Geometry check sheet. Reference: the model listing, model coordinates, mm. Face numbers are marked on the shaded views. A direction names the side the tool comes from. Round coordinates to 2 decimals unless told otherwise and drop trailing zeros. Loops run counter-clockwise (first coordinate to the right, second up) from the corner with the lowest first, then second, coordinate; pieces in that order, holes last.
```python
from build123d import *

# Parameters (mm, degrees)
SKETCH_1_R      = 118.75
EXTRUDE_1_DEPTH = 50
SKETCH_2_R      = 12.5
EXTRUDE_2_DEPTH = 10


with BuildPart() as part:
    # 草圖1 → 填料-伸長1 (new body)
    with BuildSketch(Plane(origin=(0, 0, 0), x_dir=(1, 0, 0), z_dir=(0, 1, 0))):
        Polygon((98.75, 128.75), (128.75, 98.75), (128.75, -98.75), (98.75, -128.75), (-98.75, -128.75), (-128.75, -98.75), (-128.75, 98.75), (-98.75, 128.75), align=None)
        with Locations(Location((0, 0, 0), (0, 0, 270))):
            Circle(SKETCH_1_R, mode=Mode.SUBTRACT)
    extrude(amount=EXTRUDE_1_DEPTH)

    # 草圖2 → 填料-伸長2 (add)
    with BuildSketch(Plane.XZ):
        Polygon((98.75, -128.75), (128.75, -98.75), (128.75, 98.75), (98.75, 128.75), (-98.75, 128.75), (-128.75, 98.75), (-128.75, -98.75), (-98.75, -128.75), align=None)
        with Locations(Location((0, 0, 0), (0, 0, 270))):
            Circle(SKETCH_2_R, mode=Mode.SUBTRACT)
    extrude(amount=-EXTRUDE_2_DEPTH)


solid = part.part
```
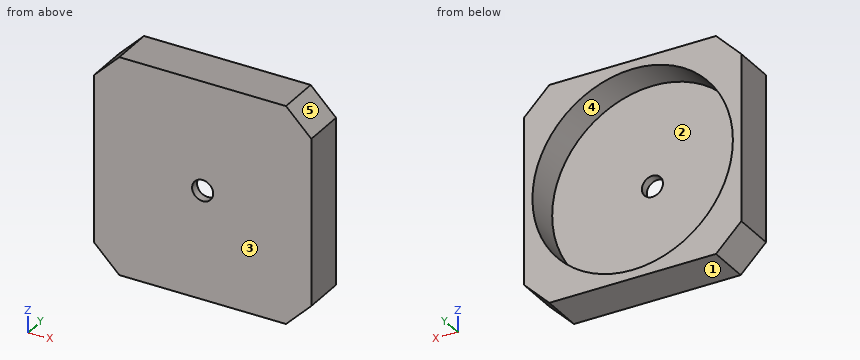
1) Sectioned sample at B-B, the plane z = 0. Record the cut outline in (x, y), then the cut area to 4 significant figures.
Report:
outline: (-128.75, 0) - (-12.5, 0) - (-12.5, 10) - (-118.75, 10) - (-118.75, 50) - (-128.75, 50) - close; (12.5, 0) - (128.75, 0) - (128.75, 50) - (118.75, 50) - (118.75, 10) - (12.5, 10) - close
area: 3,125 mm2
2) Mould release check, pull along Z, two halves, no side actions. Record for the marked faces 3, 4 and 5: +Z half, -Z half, draft (parallel to the pull), parting line (faces both ways), or undercut.
Report:
face 3: draft
face 4: undercut
face 5: +Z half
3) Sectioned sample at C-C, the plane y = 13. Record the cut outline in (x, z), then the cut area to 3 significant figures.
Report:
outline: (-128.75, -98.75) - (-98.75, -128.75) - (98.75, -128.75) - (128.75, -98.75) - (128.75, 98.75) - (98.75, 128.75) - (-98.75, 128.75) - (-128.75, 98.75) - close; hole circle Ø237.5 at (0, 0)
area: 20,200 mm2
4) Gauge pin test, flat ends, axial feed: pin 1 (5 mm diameter, centred on x = 58, z = -52.5, fed in from -Y); pin 2 (6 mm diameter, centred on x = -12, z = 63.5, fed in from +Y). Record the tip position at first contact, or that the pin passes through.
Report:
pin 1: stops at y = 0
pin 2: stops at y = 10
5) Sectioned sample at A-A, the plane x = 0. Record the cut outline in (y, z).
Report:
outline: (0, -128.75) - (50, -128.75) - (50, -118.75) - (10, -118.75) - (10, -12.5) - (0, -12.5) - close; (0, 12.5) - (10, 12.5) - (10, 118.75) - (50, 118.75) - (50, 128.75) - (0, 128.75) - close
6) Sectioned sample at D-D, the plane z = 54. Record the cut outline in (x, y).
Report:
outline: (-128.75, 0) - (128.75, 0) - (128.75, 50) - (105.76, 50) - (105.76, 10) - (-105.76, 10) - (-105.76, 50) - (-128.75, 50) - close
7) Scan lines: line 1 along Z through (x, y) = (0, 39); line 2 along X through (y, z) = (47.5, 22); line 3 along Z through (x, y) = (64.5, 35.5). Record each from-to range of solid material in increasing order.
Report:
line 1: z = -128.75 to -118.75, 118.75 to 128.75
line 2: x = -128.75 to -116.69, 116.69 to 128.75
line 3: z = -128.75 to -99.71, 99.71 to 128.75
8) Access from +Z, -Z, +X, -X, +Y, -Y to the whole of each face (thin tool, end or side, straight path). Record for the marked faces 1 and 2.
Report:
face 1: -Z, +X, -X, +Y, -Y
face 2: +Y
